Work out the finished part from the listing and answer in its coordinate system (mm). Round coordinates to 2 decimals unless told otherwise and drop trailing zeros. Order: outer loops, then holes, each group sorted by start corner. A loop starts at its lowest first (then second) coordinate and runs counter-clockwise, first axis right, second up. Notation, with made-up numbers: (77, 50) - (109, 50) arc R28 cw to (109, 85) - close; hole circle Ø10 at (54.25, 48). An arc over 180 degrees is marked (long way). Answer in a Markdown table with one row per item.
from build123d import *

# Parameters (mm, degrees)
F0_R     = 12.7
F0_R_2   = 44.45
F1_DEPTH = 6.35
F2_R     = 38.1


with BuildPart() as f1:
    # F0 (on Top) → F1 (new body)
    with BuildSketch(Plane.XY):
        with BuildLine():
            ThreePointArc((-58.0380028326, -25.7650970735), (-63.5, 0), (-58.0380028326, 25.7650970735))
            ThreePointArc((-58.0380028326, 25.7650970735), (-108.3412309289, 0), (-58.0380028326, -25.7650970735))
        make_face()
        with Locations((-76.5912309289, 0)):
            Circle(F0_R, mode=Mode.SUBTRACT)
        with BuildLine():
            ThreePointArc((57.94375, -25.976370723), (62.0954029096, -13.2819779212), (63.5, 0))
            ThreePointArc((63.5, 0), (62.0954029096, 13.2819779212), (57.94375, 25.976370723))
            ThreePointArc((57.94375, 25.976370723), (-0.1156721136, 63.4998946453), (-58.0380028326, 25.7650970735))
            ThreePointArc((-58.0380028326, 25.7650970735), (-63.5, 0), (-58.0380028326, -25.7650970735))
            ThreePointArc((-58.0380028326, -25.7650970735), (-0.1156721136, -63.4998946453), (57.94375, -25.976370723))
        make_face()
        Circle(F0_R_2, mode=Mode.SUBTRACT)
        with BuildLine():
            ThreePointArc((57.94375, 25.976370723), (62.0954029096, 13.2819779212), (63.5, 0))
            ThreePointArc((63.5, 0), (62.0954029096, -13.2819779212), (57.94375, -25.976370723))
            ThreePointArc((57.94375, -25.976370723), (107.95, 0), (57.94375, 25.976370723))
        make_face()
        with BuildLine():
            ThreePointArc((63.5, 0), (76.2, 12.7), (88.9, 0))
            ThreePointArc((88.9, 0), (76.2, -12.7), (63.5, 0))
        make_face(mode=Mode.SUBTRACT)
    extrude(amount=F1_DEPTH)

    # F2
    f2_edges = [f1.edges().sort_by_distance(p)[0] for p in [
        (-58.038003, 25.765097, 3.175),
        (57.94375, -25.976371, 3.175),
        (-58.038003, -25.765097, 3.175),
        (57.94375, 25.976371, 3.175),
    ]]
    fillet(f2_edges, radius=F2_R)


solid = f1.part
1) The mould has two halves that part along X. Classify faces 1 (the face through (0.717, 63.496, 3.131)), 2 (the face through (-64.478, 3.815, 3.131)), 3 (the face through (46, 1, 6.35)): released by +X, released by -X, zero draft, split by the parting line, or undercut.
Filled in:
| item | result |
|---|---|
| face 1 | split by the parting line |
| face 2 | undercut |
| face 3 | zero draft |
2) Find section C-C, the plane y = 19.5. Give the vertices of the cut face in (x, z), then the cut area to 3 significant figures.
Filled in:
| item | result |
|---|---|
| outline | (-101.65, 0) - (-39.94, 0) - (-39.94, 6.35) - (-101.65, 6.35) - close; (39.94, 0) - (101.26, 0) - (101.26, 6.35) - (39.94, 6.35) - close |
| area | 781 mm^2 |
3) Each of these flat-tipped pins is pushed along its axis until it touches: pin 1 (1 mm diameter, centred on y = 27, z = 5, fed in from +X); pin 2 (1.5 mm diameter, centred on y = -24.5, z = 1.5, fed in from +X); pin 3 (1.5 mm diameter, centred on y = -47.5, z = 2, fed in from -X). Where does it stop, or does it pass through?
Filled in:
| item | result |
|---|---|
| pin 1 | stops at x = 93.69 |
| pin 2 | stops at x = 97.27 |
| pin 3 | stops at x = -42.97 |
4) Find the intervals of material crossed by probe 1 along X at (y, z) = (1, 4.75); probe 2 along X at (y, z) = (-36.5, 1.5); probe 3 along Y at (x, z) = (0, 2.5), in increasing order. Write a range as from..to.
Filled in:
| item | result |
|---|---|
| probe 1 | x = -108.33..-89.25, -63.93..-44.44, 44.44..63.54, 88.86..107.93 |
| probe 2 | x = -55.31..-25.37, 25.37..55.32 |
| probe 3 | y = -63.5..-44.45, 44.45..63.5 |
5) Find section B-B, the plane y = 0. Give the vertices of the cut face in (x, z), then the cut area to 3 significant figures.
Filled in:
| item | result |
|---|---|
| outline | (-108.34, 0) - (-89.29, 0) - (-89.29, 6.35) - (-108.34, 6.35) - close; (-63.89, 0) - (-44.45, 0) - (-44.45, 6.35) - (-63.89, 6.35) - close; (44.45, 0) - (63.5, 0) - (63.5, 6.35) - (44.45, 6.35) - close; (88.9, 0) - (107.95, 0) - (107.95, 6.35) - (88.9, 6.35) - close |
| area | 486 mm^2 |
6) Find section A-A, the plane x = 0. Give the vertices of the cut face in (y, z), then the cut area to 3 significant figures.
Filled in:
| item | result |
|---|---|
| outline | (-63.5, 0) - (-44.45, 0) - (-44.45, 6.35) - (-63.5, 6.35) - close; (44.45, 0) - (63.5, 0) - (63.5, 6.35) - (44.45, 6.35) - close |
| area | 242 mm^2 |
7) Find section D-D, the plane z = 3.75. Give the number of separate pieces and of enclosed holes in the cut face, then the cut area to 3 significant figures.
Filled in:
| item | result |
|---|---|
| separate pieces | 1 |
| enclosed holes | 3 |
| area | 10,800 mm^2 |
